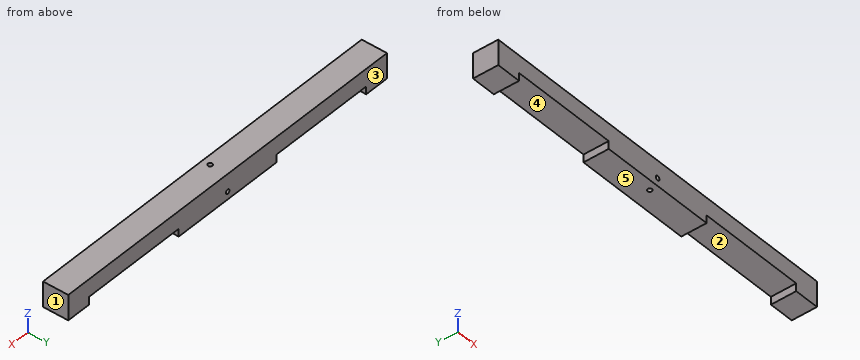
```python
from build123d import *

# Parameters (mm, degrees)
F0_W     = 26
F0_H     = 26
F1_DEPTH = 195.5
F3_W     = 110
F3_H     = 8
F4_DEPTH = 26
F6_D     = 4.5
F8_D     = 4.5


# Not quite as in the source:
# - a pattern or mirror of a feature is missing from the dataset's text; its kind, count and spacing are read off the source's solid


with BuildPart() as f1:
    # F0 (on Right) → F1 (new body, symmetric)
    with BuildSketch(Plane.YZ):
        with Locations((0, 13)):
            Rectangle(F0_W, F0_H)
    extrude(amount=F1_DEPTH, both=True)

    # F3 (on face) → F4 (cut, through all)
    with BuildSketch(Plane.XZ.offset(13)):
        with Locations((-115, 4)):
            Rectangle(F3_W, F3_H)
    f4 = extrude(amount=-F4_DEPTH, mode=Mode.SUBTRACT)

    # F4_copies: F4 across plane
    add(f4.mirror(Plane(origin=(0, 0, 0), x_dir=(0, 0, 1), z_dir=(1, 0, 0))), mode=Mode.SUBTRACT)

    # F6 (through all)
    with Locations(Plane.XZ.offset(13)):
        with Locations((0, 8)):
            Hole(F6_D / 2)

    # F8 (through all)
    with Locations(Plane.XY.offset(26)):
        with Locations((0, -5)):
            Hole(F8_D / 2)


solid = f1.part
```
Verification items for the finished model (mm, model axes). Face numbers are marked on the shaded views. A direction names the side the tool comes from. Coordinates: 2 decimals unless noted, no trailing zeros. Order: outer loops, then holes, each group sorted by start corner. A loop starts at its lowest first (then second) coordinate and runs counter-clockwise, first axis right, second up. Notation, with made-up numbers: (3.25, -18.75) -> (59.25, -18.75) arc R30 ccw to (59.25, 11.25) -> close; hole circle Ø6 at (25, 55.5). An arc over 180 degrees is marked (long way). Answer as CSV lines item,"result". Start each with the question number.
1) Gauge pin test, flat end, axial feed: pin 1 Ø4 at (x, y) = (133.5, 5) entering from -Z. Record the tip position at first contact, or that the pin passes through.
2) Release check for a two-part mould opening along X. For the marked faces 1, 2 and 3 record: released by +X, released by -X, zero draft, split by the parting line, or undercut.
3) Set-up check for the marked faces 4 and 5: record each of +Z, -Z, +X, -X, +Y, -Y from which the full face is reachable in a straight line by a thin tool's end or side.
4) Cross-section at B-B, the plane x = -141.5. Record the boundary of the cut face in (y, z).
5) Material ranges on L1, parallel to X at y = 5.5, z = 5.5; L2, parallel to X at y = -5, z = 5.75; L3, parallel to Y at x = 0, z = 20, recorded low to high. Write a range as [from, to].
6) Cross-section at A-A, the plane y = 9. Record the boundary of the cut face in (x, z).
Conclusion:
1,pin 1,"stops at z = 8"
2,face 1,"released by +X"
2,face 2,"undercut"
2,face 3,"zero draft"
3,face 4,"-Z, +Y, -Y"
3,face 5,"-Z, +X, -X, +Y, -Y"
4,outline,"(-13, 8) -> (13, 8) -> (13, 26) -> (-13, 26) -> close"
5,L1,"x = [-195.5, -170], [-60, 60], [170, 195.5]"
5,L2,"x = [-195.5, -170], [-60, -2.25], [2.25, 60], [170, 195.5]"
5,L3,"y = [-13, -7.25], [-2.75, 13]"
6,outline,"(-195.5, 0) -> (-170, 0) -> (-170, 8) -> (-60, 8) -> (-60, 0) -> (60, 0) -> (60, 8) -> (170, 8) -> (170, 0) -> (195.5, 0) -> (195.5, 26) -> (-195.5, 26) -> close; hole circle Ø4.5 at (0, 8)"
